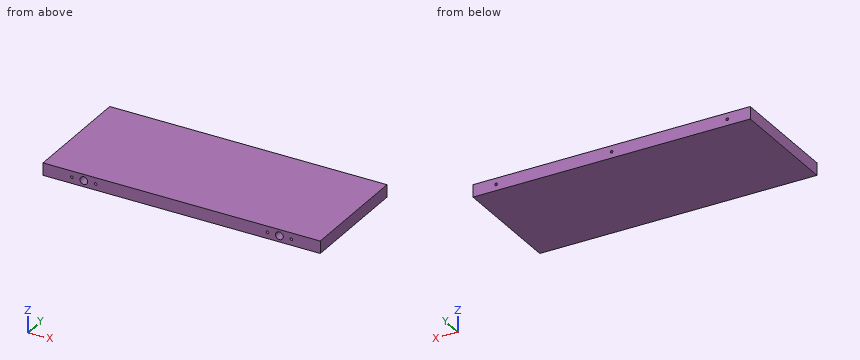
from build123d import *

# Parameters (mm, degrees)
SKETCH1_W                      = 360
SKETCH1_H                      = 150
BOSS_EXTRUDE1_DEPTH            = 8
F_8_36_TAPPED_HOLE1_AT_2_COUNT = 2
F_8_36_TAPPED_HOLE1_AT_2_PITCH = 31
F_8_36_TAPPED_HOLE2_D          = 3.4544
F_8_36_TAPPED_HOLE2_DEPTH      = 25
F_8_36_TAPPED_HOLE2_TIP        = 1.037806461


with BuildPart() as part:
    # Sketch1 → Boss-Extrude1 (new, symmetric)
    with BuildSketch(Plane.XY):
        Rectangle(SKETCH1_W, SKETCH1_H)
    extrude(amount=BOSS_EXTRUDE1_DEPTH, both=True)

    # Sketch3 → #8-36 Tapped Hole1 (revolve, cut)
    with BuildSketch(Plane(origin=(-142.5, -75, 0), x_dir=(0, 0, -1), z_dir=(1, 0, 0))):
        Polygon((0, 0), (0, 26.037806461), (1.7272, 25), (1.7272, 0), align=None)
    f_8_36_tapped_hole1 = revolve(axis=Axis((-142.5, -81.35, 0), (0, 1, 0)), mode=Mode.SUBTRACT)

    # #8-36 Tapped Hole1 at 2: #8-36 Tapped Hole1 ×2
    with Locations(*[(i * F_8_36_TAPPED_HOLE1_AT_2_PITCH, 0, 0) for i in range(1, F_8_36_TAPPED_HOLE1_AT_2_COUNT)]):
        add(f_8_36_tapped_hole1, mode=Mode.SUBTRACT)

    # Sketch6 → M8 Clearance Hole1 (revolve, cut)
    with BuildSketch(Plane(origin=(-127, -75, 0), x_dir=(0, 0, -1), z_dir=(1, 0, 0))):
        Polygon((0, 0), (0, 48.004303095), (5, 45), (5, 0), align=None)
    m8_clearance_hole1 = revolve(axis=Axis((-127, -81.35, 0), (0, 1, 0)), mode=Mode.SUBTRACT)

    # Mirror1: #8-36 Tapped Hole1, M8 Clearance Hole1 across plane
    add(f_8_36_tapped_hole1.mirror(Plane(origin=(0, 0, 0), x_dir=(0, 0, 1), z_dir=(1, 0, 0))), mode=Mode.SUBTRACT)
    add(m8_clearance_hole1.mirror(Plane(origin=(0, 0, 0), x_dir=(0, 0, 1), z_dir=(1, 0, 0))), mode=Mode.SUBTRACT)

    # Mirror1 copy 1 sketch → Mirror1 copy 1 (revolve, cut)
    with BuildSketch(Plane(origin=(111.5, -75, 0), x_dir=(0, 0, -1), z_dir=(-1, 0, 0))):
        Polygon((0, 0), (0, -26.037806461), (1.7272, -25), (1.7272, 0), align=None)
    revolve(axis=Axis((111.5, -81.35, 0), (0, -1, 0)), mode=Mode.SUBTRACT)

    # #8-36 Tapped Hole2
    with Locations(Plane(origin=(597.704940286, 75, -222), x_dir=(1, 0, 0), z_dir=(0, 1, 0))):
        with Locations((-447.704940286, -222), (-597.704940286, -222), (-747.704940286, -222)):
            Hole(F_8_36_TAPPED_HOLE2_D / 2, depth=F_8_36_TAPPED_HOLE2_DEPTH)
            with Locations((0, 0, -(F_8_36_TAPPED_HOLE2_DEPTH + F_8_36_TAPPED_HOLE2_TIP / 2))):  # 118° drill point
                Cone(0, F_8_36_TAPPED_HOLE2_D / 2, F_8_36_TAPPED_HOLE2_TIP, mode=Mode.SUBTRACT)


solid = part.part
For this review, take the finished solid that the model builds, in its own axes (mm). Give positions to 0.01 mm unless a question says otherwise; leave off trailing zeros. Order: outer loops, then holes, each group sorted by start corner. A loop starts at its lowest first (then second) coordinate and runs counter-clockwise, first axis right, second up. Notation, with made-up numbers: M 77.5,4.25 L 124.5,4.25 A24 cw 124.5,43.25 Z; hole C 67,-37 d10. An arc over 180 degrees is marked long. Answer in a Markdown table with one row per item. Add a question column.
(1) Consider section A-A on y = -44. State the section outline as (x, z) points.
(2) Wall thickness on probe 1 along Z at (x, y) = (-111.5, -62.5); probe 2 along X at (y, z) = (-65.5, 2.75); probe 3 along Z at (x, y) = (-127, -56.5): over which ranges is each line inside the solid? List them lowest first. Write a range as [from, to].
(3) For pin 1 (2 mm diameter, centred on x = 150, z = 0, fed in from +Y), flat-tipped, find the tip position at first contact; note if it passes through.
Evaluation:
| question | item | result |
|---|---|---|
| 1 | outline | M -180,-8 L 180,-8 L 180,8 L -180,8 Z; hole C -127,0 d10; hole C 127,0 d10 |
| 2 | probe 1 | z = [-8, -1.73], [1.73, 8] |
| 2 | probe 2 | x = [-180, -131.18], [-122.82, 122.82], [131.18, 180] |
| 2 | probe 3 | z = [-8, -5], [5, 8] |
| 3 | pin 1 | stops at y = 49.56 |
